```python
from build123d import *

# Parameters (mm, degrees)
BOSS_EXTRUDE1_DEPTH     = 10
BOSS_EXTRUDE6_DEPTH     = 41
CUT_EXTRUDE1_REACH      = 80.865
CUT_EXTRUDE2_REACH      = 80.865
BOSS_EXTRUDE9_DEPTH     = 10
CHAMFER3_SIZE           = 10
CUT_EXTRUDE3_DEPTH      = 77.842469388
CUT_EXTRUDE3_DEPTH_BACK = 77.842469388
BOSS_EXTRUDE10_DEPTH    = 55.25
SKETCH13_W              = 20
SKETCH13_H              = 5
BOSS_EXTRUDE11_DEPTH    = 92.85
CUT_EXTRUDE4_REACH      = 147.324
SKETCH14_R              = 2
SKETCH15_W              = 15
SKETCH15_H              = 5
BOSS_EXTRUDE12_DEPTH    = 28.25
FILLET1_R               = 10
CHAMFER4_SIZE           = 10


with BuildPart() as part:
    # Sketch2 → Boss-Extrude1 (new body)
    with BuildSketch(Plane.XY):
        Polygon((-5, -50.944473192), (-5, -0.20517252), (44.083730464, 1.808954014), (44.083730464, -29.38936641), (24.227900916, -50.944473192), align=None)
    extrude(amount=BOSS_EXTRUDE1_DEPTH)

    # Sketch2<5> → Boss-Extrude6 (add)
    with BuildSketch(Plane.XY):
        Polygon((-5, -0.20517252), (-5, -50.944473192), (24.227900916, -50.944473192), (28.833730464, -45.944473192), (0, -45.944473192), (0, 0), align=None)
    extrude(amount=-BOSS_EXTRUDE6_DEPTH)

    # Sketch6 → Cut-Extrude1 (cut, up to next)
    with BuildSketch(Plane(origin=(0, 0, 0), x_dir=(0, 0, -1), z_dir=(1, 0, 0)), mode=Mode.PRIVATE) as cut_extrude1_sk1:
        with BuildLine():
            Line((31.5, 0), (31.5, -33.944473192))
            ThreePointArc((31.5, -33.944473192), (47.717514421, -40.661987613), (41, -24.444473192))
            Line((41, -24.444473192), (41, 0))
            Line((41, 0), (31.5, 0))
        make_face()
    cut_extrude1_tool1 = extrude(cut_extrude1_sk1.sketch, amount=-CUT_EXTRUDE1_REACH, mode=Mode.PRIVATE) & part.part
    add(cut_extrude1_tool1.solids().sort_by_distance((0, -24.250765, -38.671635))[0], mode=Mode.SUBTRACT)

    # Sketch7 → Cut-Extrude2 (cut, up to next)
    with BuildSketch(Plane(origin=(0, 0, 0), x_dir=(-1, 0, 0), z_dir=(0, 0, -1)), mode=Mode.PRIVATE) as cut_extrude2_sk1:
        Polygon((-5, -4.799035286), (-39.083730464, -3.400426311), (-39.083730464, -27.437423368), (-26.641496625, -40.944473192), (-5, -40.944473192), align=None)
    cut_extrude2_tool1 = extrude(cut_extrude2_sk1.sketch, amount=-CUT_EXTRUDE2_REACH, mode=Mode.PRIVATE) & part.part
    add(cut_extrude2_tool1.solids().sort_by_distance((21.232744, -21.521517, 0))[0], mode=Mode.SUBTRACT)

    # Sketch10 → Boss-Extrude9 (add)
    with BuildSketch(Plane.XY.offset(-28.5)):
        Polygon((28.833730464, -45.944473192), (0, -45.944473192), (0, 0), (10, 0.41034504), (10, -35.944473192), (28.833730464, -35.944473192), align=None)
    extrude(amount=BOSS_EXTRUDE9_DEPTH)

    # Chamfer3
    chamfer3_edges = [part.edges().sort_by_distance(p)[0] for p in [
        (19.416865232, -35.944473192, -18.5),
        (10, -17.767064076, -18.5),
    ]]
    chamfer(chamfer3_edges, length=CHAMFER3_SIZE - 0.0001)  # a hair under: the kernel refuses the full size

    # Sketch11 → Cut-Extrude3 (cut, two sides: drawn at the far end of the back side and taken through both)
    with BuildSketch(Plane(origin=(0, -45.944473192, 0), x_dir=(1, 0, 0), z_dir=(0, 1, 0)).offset(-CUT_EXTRUDE3_DEPTH_BACK)):
        Polygon((28.833730464, 41), (16.833730464, 41), (28.833730464, 0), align=None)
    extrude(amount=CUT_EXTRUDE3_DEPTH + CUT_EXTRUDE3_DEPTH_BACK, mode=Mode.SUBTRACT)

    # Sketch12 → Boss-Extrude10 (add)
    with BuildSketch(Plane(origin=(0, 0, -41), x_dir=(-1, 0, 0), z_dir=(0, 0, -1))):
        Polygon((0, -45.944473192), (-16.833730464, -45.944473192), (-16.833730464, -50.944473192), (5, -50.944473192), (5, -43.444473192), (0, -43.444473192), align=None)
    extrude(amount=BOSS_EXTRUDE10_DEPTH)

    # Sketch13 → Boss-Extrude11 (add)
    with BuildSketch(Plane.ZY.offset(5)):
        with Locations((-58, -48.444473192)):
            Rectangle(SKETCH13_W, SKETCH13_H)
    extrude(amount=BOSS_EXTRUDE11_DEPTH)

    # Sketch14 → Cut-Extrude4 (cut, up to next)
    with BuildSketch(Plane(origin=(0, -45.944473192, 0), x_dir=(1, 0, 0), z_dir=(0, 1, 0)), mode=Mode.PRIVATE) as cut_extrude4_sk1:
        with Locations(Location((-87.85, 58, 0), (0, 0, 270))):
            Circle(SKETCH14_R)
    cut_extrude4_tool1 = extrude(cut_extrude4_sk1.sketch, amount=-CUT_EXTRUDE4_REACH, mode=Mode.PRIVATE) & part.part
    add(cut_extrude4_tool1.solids().sort_by_distance((-87.85, -45.944473, -58))[0], mode=Mode.SUBTRACT)

    # Sketch15 → Boss-Extrude12 (add)
    with BuildSketch(Plane(origin=(0, 0, -68), x_dir=(-1, 0, 0), z_dir=(0, 0, -1))):
        with Locations((78.35, -48.444473192)):
            Rectangle(SKETCH15_W, SKETCH15_H)
    extrude(amount=BOSS_EXTRUDE12_DEPTH)

    # Mirror1: part across plane


with BuildPart() as part_1:
    add(part.part)
    add(part.part.mirror(Plane(origin=(0, 0, -96.25), x_dir=(1, 0, 0), z_dir=(0, 0, -1))))

    # Fillet1
    fillet1_edges = [part_1.edges().sort_by_distance(p)[0] for p in [
        (-97.85, -48.444473192, -144.5),
        (-97.85, -48.444473192, -48),
        (-97.85, -48.444473192, -124.5),
        (-97.85, -48.444473192, -68),
    ]]
    fillet(fillet1_edges, radius=FILLET1_R - 0.0001)  # a hair under: the kernel refuses the full size

    # Chamfer4
    chamfer4_edges = [part_1.edges().sort_by_distance(p)[0] for p in [
        (-5, -48.444473192, -68),
        (-5, -48.444473192, -48),
        (-70.85, -48.444473192, -68),
        (-70.85, -48.444473192, -124.5),
        (-5, -48.444473192, -124.5),
        (-5, -48.444473192, -144.5),
    ]]
    chamfer(chamfer4_edges, length=CHAMFER4_SIZE)


solid = part_1.part
```
Geometry: final body of the model. Coordinates: model frame, mm. A direction names the side the tool comes from. Give positions to 0.01 mm unless a question says otherwise; leave off trailing zeros. Loops run counter-clockwise (first coordinate to the right, second up) from the corner with the lowest first, then second, coordinate; pieces in that order, holes last. Notation, with made-up numbers: (38.5, 61.5) -> (63.5, 61.5) arc R28 cw to (63.5, 98.5) -> close; hole circle Ø7 at (33, 6.25). An arc over 180 degrees is marked (long way). Return JSON: item names as keys, results as strings.
Item 1: Section B-B, the plane x = -77. Output: boundary loops of the cut face in (y, z), plus the area to 4 significant figures.
Filled in:
{"outline": "(-50.94, -144.5) -> (-45.94, -144.5) -> (-45.94, -48) -> (-50.94, -48) -> close", "area": "482.5 mm^2"}
Item 2: Line query: line 1 (X direction, y = -49.5, z = -58); line 2 (Z direction, x = -1, y = -33.5); line 3 (X direction, y = -5, z = -186). Output: solid intervals per line, ascending.
Filled in:
{"line 1": "-97.85 to -89.85, -85.85 to 16.83", "line 2": "-202.5 to -161, -31.5 to 10", "line 3": "-5 to 0"}
Item 3: Section C-C, the plane z = -34. Output: boundary loops of the cut face in (x, y), plus the area to 3 significant figures.
Filled in:
{"outline": "(-5, -50.94) -> (18.88, -50.94) -> (18.88, -45.94) -> (0, -45.94) -> (0, -40.37) -> (-5, -40.37) -> close", "area": "147 mm^2"}
Item 4: Access query for faces 4 (the flat face through (-10.1, -48.5, -119.6)), 5 (the flat face through (32.95, -34.096, 4.93)), 6 (the flat face through (15, -45.944, -9)), 7 (the flat face through (-51, -48, -144.5)). Directions: +Z, -Z, +X, -X, +Y, -Y. A direction counts if a zero-diameter tool reaches every point of the face in a straight line with its end or side. Return the directions, or none.
Filled in:
{"face 4": "+Y, -Y", "face 5": "+Z, -Z", "face 6": "+X, +Y", "face 7": "-Z, -X, +Y, -Y"}
Item 5: Mould query, pull axis Z, two halves, no side actions, for faces 1 (the flat face through (-65.78, -48.48, -72.93)), 2 (the cylindrical face through (-94.84, -48.41, -141.65)), 3 (the flat face through (39.084, -15, 5)). Classes: released by +Z, released by -Z, zero draft, split by the parting line, or undercut.
Filled in:
{"face 1": "undercut", "face 2": "released by -Z", "face 3": "zero draft"}
Item 6: Pin query (flat end, axial travel): P1, Ø5.5, axis at x = -3.5, z = -103.5, coming from the +Y side; P2, Ø1.5, axis at y = -49, z = -88, coming from the -X side; P3, Ø9.5, axis at x = 17.5, z = -7, coming from the +Y side. Return the tip coordinate at first contact, or that it passes through.
Filled in:
{"P1": "y = -43.44", "P2": "x = -85.85", "P3": "y = -45.94"}
Item 7: Section A-A, the plane y = -8.5. Count the separate pieces of the cut face and the enclosed holes in it, plus the area to 3 significant figures.
Filled in:
{"separate pieces": "4", "enclosed holes": "0", "area": "715 mm^2"}
